from build123d import *

# Parameters (mm, degrees)
CYLINDER032_R           = 2
CYLINDER032_DEPTH       = 2
CYLINDER032_PITCH_ANGLE = 90
CYLINDER033_R           = 2
CYLINDER033_DEPTH       = 2
CYLINDER033_PITCH_ANGLE = 90
CYLINDER030_R           = 1
CYLINDER030_DEPTH       = 7
CYLINDER030_PITCH_ANGLE = 90
CYLINDER031_R           = 1
CYLINDER031_DEPTH       = 7
CYLINDER031_PITCH_ANGLE = 90
CYLINDER029_R           = 2
CYLINDER029_DEPTH       = 7
CYLINDER029_PITCH_ANGLE = 90
CYLINDER028_R           = 2
CYLINDER028_DEPTH       = 7
CYLINDER028_PITCH_ANGLE = 90
CYLINDER027_R           = 2
CYLINDER027_DEPTH       = 2
CYLINDER027_PITCH_ANGLE = 90
CYLINDER026_R           = 1
CYLINDER026_DEPTH       = 10
CYLINDER026_PITCH_ANGLE = 90
CYLINDER024_R           = 2
CYLINDER024_DEPTH       = 10
CYLINDER024_PITCH_ANGLE = 90
CYLINDER025_R           = 2
CYLINDER025_DEPTH       = 10
CYLINDER025_PITCH_ANGLE = 90
BOX038_W                = 7
BOX038_H                = 20
BOX038_DEPTH            = 54
FILLET010_R             = 5
CHAMFER019_SIZE         = 2


with BuildPart() as cylinder032:
    # Cylinder032 → Cylinder032 (new body)
    with BuildSketch(Plane.XY):
        Circle(CYLINDER032_R)
    extrude(amount=CYLINDER032_DEPTH)


with BuildPart() as cylinder032_1:
    # Cylinder032 pitch: moved
    add(cylinder032.part.rotate(Axis((0, 0, 0), (0, 1, 0)), CYLINDER032_PITCH_ANGLE))


with BuildPart() as cylinder032_2:
    # Cylinder032 placement: moved
    add(cylinder032_1.part.moved(Location((-2, -42, -12.3))))


with BuildPart() as cylinder033:
    # Cylinder033 → Cylinder033 (new body)
    with BuildSketch(Plane.XY):
        Circle(CYLINDER033_R)
    extrude(amount=CYLINDER033_DEPTH)


with BuildPart() as cylinder033_1:
    # Cylinder033 pitch: moved
    add(cylinder033.part.rotate(Axis((0, 0, 0), (0, 1, 0)), CYLINDER033_PITCH_ANGLE))


with BuildPart() as cylinder033_2:
    # Cylinder033 placement: moved
    add(cylinder033_1.part.moved(Location((-2, -42, 24.7))))


with BuildPart() as cylinder030:
    # Cylinder030 → Cylinder030 (new body)
    with BuildSketch(Plane.XY):
        Circle(CYLINDER030_R)
    extrude(amount=CYLINDER030_DEPTH)


with BuildPart() as cylinder030_1:
    # Cylinder030 pitch: moved
    add(cylinder030.part.rotate(Axis((0, 0, 0), (0, 1, 0)), CYLINDER030_PITCH_ANGLE))


with BuildPart() as cylinder030_2:
    # Cylinder030 placement: moved
    add(cylinder030_1.part.moved(Location((-7, -42, -12.3))))


with BuildPart() as cylinder031:
    # Cylinder031 → Cylinder031 (new body)
    with BuildSketch(Plane.XY):
        Circle(CYLINDER031_R)
    extrude(amount=CYLINDER031_DEPTH)


with BuildPart() as cylinder031_1:
    # Cylinder031 pitch: moved
    add(cylinder031.part.rotate(Axis((0, 0, 0), (0, 1, 0)), CYLINDER031_PITCH_ANGLE))


with BuildPart() as cylinder031_2:
    # Cylinder031 placement: moved
    add(cylinder031_1.part.moved(Location((-7, -42, 24.7))))


with BuildPart() as cylinder029:
    # Cylinder029 → Cylinder029 (new body)
    with BuildSketch(Plane.XY):
        Circle(CYLINDER029_R)
    extrude(amount=CYLINDER029_DEPTH)


with BuildPart() as cylinder029_1:
    # Cylinder029 pitch: moved
    add(cylinder029.part.rotate(Axis((0, 0, 0), (0, 1, 0)), CYLINDER029_PITCH_ANGLE))


with BuildPart() as cylinder029_2:
    # Cylinder029 placement: moved
    add(cylinder029_1.part.moved(Location((-7, -42, 24.7))))


with BuildPart() as cylinder028:
    # Cylinder028 → Cylinder028 (new body)
    with BuildSketch(Plane.XY):
        Circle(CYLINDER028_R)
    extrude(amount=CYLINDER028_DEPTH)


with BuildPart() as cylinder028_1:
    # Cylinder028 pitch: moved
    add(cylinder028.part.rotate(Axis((0, 0, 0), (0, 1, 0)), CYLINDER028_PITCH_ANGLE))


with BuildPart() as cylinder028_2:
    # Cylinder028 placement: moved
    add(cylinder028_1.part.moved(Location((-7, -42, -12.3))))


with BuildPart() as cylinder027:
    # Cylinder027 → Cylinder027 (new body)
    with BuildSketch(Plane.XY):
        Circle(CYLINDER027_R)
    extrude(amount=CYLINDER027_DEPTH)


with BuildPart() as cylinder027_1:
    # Cylinder027 pitch: moved
    add(cylinder027.part.rotate(Axis((0, 0, 0), (0, 1, 0)), CYLINDER027_PITCH_ANGLE))


with BuildPart() as cylinder027_2:
    # Cylinder027 placement: moved
    add(cylinder027_1.part.moved(Location((-7, -42, 6))))


with BuildPart() as cylinder026:
    # Cylinder026 → Cylinder026 (new body)
    with BuildSketch(Plane.XY):
        Circle(CYLINDER026_R)
    extrude(amount=CYLINDER026_DEPTH)


with BuildPart() as cylinder026_1:
    # Cylinder026 pitch: moved
    add(cylinder026.part.rotate(Axis((0, 0, 0), (0, 1, 0)), CYLINDER026_PITCH_ANGLE))


with BuildPart() as cylinder026_2:
    # Cylinder026 placement: moved
    add(cylinder026_1.part.moved(Location((-7, -42, 6))))


with BuildPart() as cylinder024:
    # Cylinder024 → Cylinder024 (new body)
    with BuildSketch(Plane.XY):
        Circle(CYLINDER024_R)
    extrude(amount=CYLINDER024_DEPTH)


with BuildPart() as cylinder024_1:
    # Cylinder024 pitch: moved
    add(cylinder024.part.rotate(Axis((0, 0, 0), (0, 1, 0)), CYLINDER024_PITCH_ANGLE))


with BuildPart() as cylinder024_2:
    # Cylinder024 placement: moved
    add(cylinder024_1.part.moved(Location((-8, -42, 24.7))))


with BuildPart() as cylinder025:
    # Cylinder025 → Cylinder025 (new body)
    with BuildSketch(Plane.XY):
        Circle(CYLINDER025_R)
    extrude(amount=CYLINDER025_DEPTH)


with BuildPart() as cylinder025_1:
    # Cylinder025 pitch: moved
    add(cylinder025.part.rotate(Axis((0, 0, 0), (0, 1, 0)), CYLINDER025_PITCH_ANGLE))


with BuildPart() as cylinder025_2:
    # Cylinder025 placement: moved
    add(cylinder025_1.part.moved(Location((-8, -42, -12.3))))


with BuildPart() as cut046:
    # Box038 → Box038 (new body)
    with BuildSketch(Plane(origin=(-7, -52, -20.8), x_dir=(1, 0, 0), z_dir=(0, 0, 1))):
        with Locations((3.5, 10)):
            Rectangle(BOX038_W, BOX038_H)
    extrude(amount=BOX038_DEPTH)

    # Fillet010
    fillet010_edges = [cut046.edges().sort_by_distance(p)[0] for p in [
        (-3.5, -52, -20.8),
        (-3.5, -52, 33.2),
        (-3.5, -32, -20.8),
        (-3.5, -32, 33.2),
    ]]
    fillet(fillet010_edges, radius=FILLET010_R)

    # Chamfer019
    chamfer019_edges = [cut046.edges().sort_by_distance(p)[0] for p in [
        (0, -42, -20.8),
    ]]
    chamfer(chamfer019_edges, length=CHAMFER019_SIZE)

    # Cut038: cut Cylinder025
    add(cylinder025_2.part, mode=Mode.SUBTRACT)

    # Cut039: cut Cylinder024
    add(cylinder024_2.part, mode=Mode.SUBTRACT)

    # Cut041: cut Cylinder026
    add(cylinder026_2.part, mode=Mode.SUBTRACT)

    # Cut042: cut Cylinder027
    add(cylinder027_2.part, mode=Mode.SUBTRACT)

    # Fusion023: union Cylinder028
    add(cylinder028_2.part)

    # Fusion024: union Cylinder029
    add(cylinder029_2.part)

    # Cut043: cut Cylinder031
    add(cylinder031_2.part, mode=Mode.SUBTRACT)

    # Cut044: cut Cylinder030
    add(cylinder030_2.part, mode=Mode.SUBTRACT)

    # Cut045: cut Cylinder033
    add(cylinder033_2.part, mode=Mode.SUBTRACT)

    # Cut046: cut Cylinder032
    add(cylinder032_2.part, mode=Mode.SUBTRACT)


solid = cut046.part
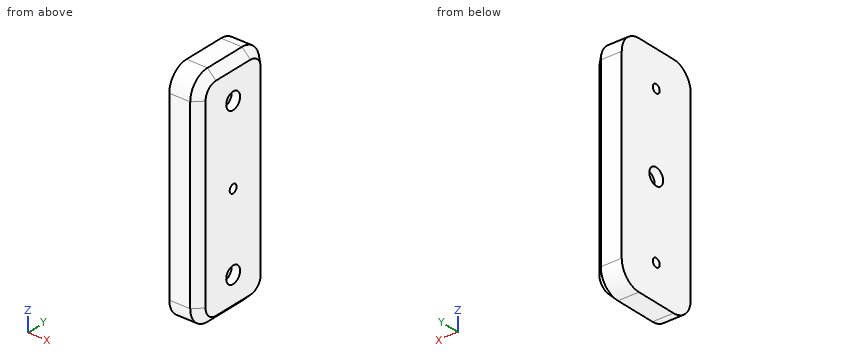
Model file for the job. Use its own axes, mm. Coordinates: 2 decimals unless noted, no trailing zeros. Write each loop counter-clockwise with the first axis right and the second up, starting at its lowest first coordinate (ties: lowest second). Pieces come first, ordered by that corner, then holes. Notation, with made-up numbers: (-28, -37.5) -> (21, -37.5) arc R16 ccw to (21, -30.5) -> close; hole circle Ø10 at (-37.5, 66). An arc over 180 degrees is marked (long way). One line per item, written item: value. Start each with the question number.
1) Slice it at A-A on y = -42. Count the separate pieces of the cut face and the enclosed holes in it, then the cut area to 3 significant figures.
2) Slice it at D-D on z = 8.5. Write the cut outline in (x, y), then the cut area to 3 significant figures.
3) Slice it at C-C on z = 24.7. Write the cut outline in (x, y).
4) Slice it at B-B on x = -1.5. Write the cut outline in (y, z), then the cut area to 3 significant figures.
5) Probe probe 1 along Z at (x, y) = (-3.1, -42); probe 2 along Y at (x, z) = (-4.35, 24.7); probe 3 along Z at (x, y) = (-5.5, -42.25). List the from-to ranges inside material, lowest first.
Answers follow:
1. separate pieces: 4
1. enclosed holes: 0
1. area: 320 mm2
2. outline: (-7, -52) -> (-2, -52) -> (0, -50) -> (0, -34) -> (-2, -32) -> (-7, -32) -> close
2. area: 136 mm2
3. outline: (-7, -52) -> (-2, -52) -> (0, -50) -> (0, -44) -> (-2, -44) -> (-2, -43) -> (-7, -43) -> close; (-7, -41) -> (-2, -41) -> (-2, -40) -> (0, -40) -> (0, -34) -> (-2, -32) -> (-7, -32) -> close
4. outline: (-51.5, -15.8) arc R4.5 ccw to (-47, -20.3) -> (-37, -20.3) arc R4.5 ccw to (-32.5, -15.8) -> (-32.5, 28.2) arc R4.5 ccw to (-37, 32.7) -> (-47, 32.7) arc R4.5 ccw to (-51.5, 28.2) -> close; hole circle Ø4 at (-42, -12.3); hole circle Ø4 at (-42, 24.7); hole circle Ø2 at (-42, 6)
4. area: 961 mm2
5. probe 1: -20.8 to -13.3, -11.3 to 5, 7 to 23.7, 25.7 to 33.2
5. probe 2: -52 to -43, -41 to -32
5. probe 3: -20.8 to -13.27, -11.33 to 4.02, 7.98 to 23.73, 25.67 to 33.2
